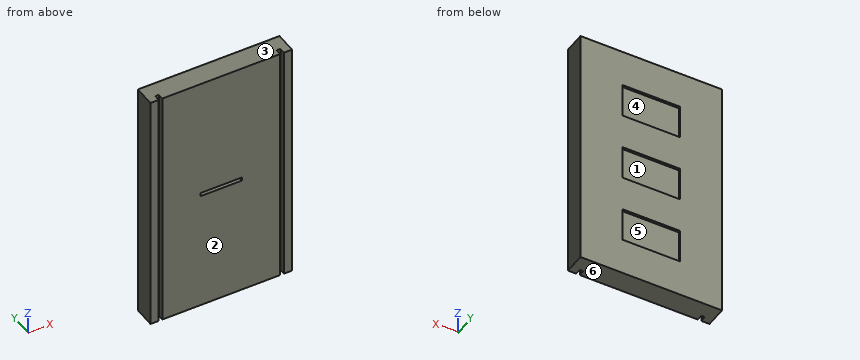
Autodesk Inventor part; units mm, degrees
ref_plane "YZ Plane" through (0, 0, 0) normal (1, 0, 0) x (0, 1, 0)
ref_plane "XZ Plane" through (0, 0, 0) normal (0, 1, 0) x (-1, 0, 0)
ref_plane "XY Plane" through (0, 0, 0) normal (0, 0, 1) x (1, 0, 0)
sketch "Sketch1" plane through (0, 0, 0) normal (0, 0, 1) x (1, 0, 0)
  line L0 (0, 0) -> (120, 0)
  line L1 (120, 0) -> (120, 18)
  line L2 (120, 18) -> (0, 18)
  line L3 (0, 18) -> (0, 0)
  dimension "d0" = 18
  dimension "d1" = 120
extrude "Extrusion1" add sketch "Sketch1" along normal blind 210
sketch "Sketch2" plane through (0, 0, 210) normal (0, 0, 1) x (1, 0, 0)
  line L0 (0, 0) -> (120, 0)
  line L1 (7, 0) -> (10, 0)
  line L2 (10, 0) -> (10, 5)
  line L3 (10, 5) -> (7, 5)
  line L4 (7, 5) -> (7, 0)
  line L5 (60, 0) -> (60, -17.5294) construction
  line L6 (113, 0) -> (110, 0)
  line L7 (110, 0) -> (110, 5)
  line L8 (110, 5) -> (113, 5)
  line L9 (113, 5) -> (113, 0)
  point P0 (110, 0)
  point P1 (113, 0)
  dimension "d4" = 3
  dimension "d5" = 5
  dimension "d26" = 100
extrude "Extrusion2" cut sketch "Sketch2" against normal through all
sketch "Sketch3" plane through (0, 18, 0) normal (0, 1, 0) x (1, 0, 0)
  line L0 (35.5, -31.5) -> (84.5, -31.5)
  line L1 (84.5, -31.5) -> (84.5, -60.5)
  line L2 (84.5, -60.5) -> (35.5, -60.5)
  line L3 (35.5, -60.5) -> (35.5, -31.5)
  line L4 (35.5, -90.5) -> (84.5, -90.5)
  line L5 (84.5, -90.5) -> (84.5, -119.5)
  line L6 (84.5, -119.5) -> (35.5, -119.5)
  line L7 (35.5, -119.5) -> (35.5, -90.5)
  line L8 (35.5, -149.5) -> (84.5, -149.5)
  line L9 (84.5, -149.5) -> (84.5, -178.5)
  line L10 (84.5, -178.5) -> (35.5, -178.5)
  line L11 (35.5, -178.5) -> (35.5, -149.5)
  line L12 (0, 0) -> (0, -210)
  line L13 (120, 0) -> (0, 0)
  point P0 (0, -105)
  point P1 (35.5, -105)
  point P2 (60, 0)
  point P3 (60, -31.5)
  dimension "d9" = 29
  dimension "d10" = 49
  dimension "d13" = 59
extrude "Extrusion3" cut sketch "Sketch3" against normal blind 2
sketch "Sketch4" plane through (10, 0, 0) normal (0, -1, 0) x (1, 0, 0)
  line L0 (-10, 0) -> (-10, 210)
  line L1 (0, 0) -> (100, 0)
  line L2 (32.5, 106.5) -> (67.5, 106.5)
  line L3 (67.5, 106.5) -> (67.5, 103.5)
  line L4 (67.5, 103.5) -> (32.5, 103.5)
  line L5 (32.5, 103.5) -> (32.5, 106.5)
  point P0 (-10, 105)
  point P1 (32.5, 105)
  point P2 (50, 103.5)
  point P3 (50, 0)
  dimension "d20" = 3
  dimension "d21" = 35
extrude "Extrusion4" cut sketch "Sketch4" against normal blind 5
properties part number "topplatform"
Design review of the part built by this model. Coordinates are the model's own, in mm. Face numbers are marked on the shaded views. A direction names the side the tool comes from. Round coordinates to 2 decimals unless told otherwise and drop trailing zeros. Order: outer loops, then holes, each group sorted by start corner. A loop starts at its lowest first (then second) coordinate and runs counter-clockwise, first axis right, second up. Notation, with made-up numbers: (15, 22.5) - (26, 22.5) arc R22 ccw to (26, 37.5) - close; hole circle Ø9 at (-22, 38.5). An arc over 180 degrees is marked (long way). Return JSON: item names as keys, results as strings.
Q1. Machinability: for the marked faces 5 and 6, which of the approach directions +Z, -Z, +X, -X, +Y, -Y give a long, thin tool a straight path to every point of the face, cutting with its end or side? Answer none if there is none.
Computed values:
{"face 5": "+Y", "face 6": "-Z, +X, -X, +Y, -Y"}
Q2. Consider section C-C on z = 55. Write out the cut boundary in (x, y).
Computed values:
{"outline": "(0, 0) - (7, 0) - (7, 5) - (10, 5) - (10, 0) - (110, 0) - (110, 5) - (113, 5) - (113, 0) - (120, 0) - (120, 18) - (84.5, 18) - (84.5, 16) - (35.5, 16) - (35.5, 18) - (0, 18) - close"}
Q3. Wall thickness on L1, parallel to X at y = 4.25, z = 92.5; L2, parallel to Z at x = 79.5, y = 16.5; L3, parallel to Z at x = 67, y = 1: over which ranges is each line inside the solid? List them lowest first. Write a range as [from, to].
Computed values:
{"L1": "x = [0, 7], [10, 110], [113, 120]", "L2": "z = [0, 31.5], [60.5, 90.5], [119.5, 149.5], [178.5, 210]", "L3": "z = [0, 103.5], [106.5, 210]"}
Q4. Consider section B-B on x = 65.5. Write out the cut boundary in (y, z).
Computed values:
{"outline": "(0, 0) - (18, 0) - (18, 31.5) - (16, 31.5) - (16, 60.5) - (18, 60.5) - (18, 90.5) - (16, 90.5) - (16, 119.5) - (18, 119.5) - (18, 149.5) - (16, 149.5) - (16, 178.5) - (18, 178.5) - (18, 210) - (0, 210) - (0, 106.5) - (5, 106.5) - (5, 103.5) - (0, 103.5) - close"}
Q5. Consider section A-A on y = 2.75. Write out the cut boundary in (x, z), plus the area to 3 significant figures.
Computed values:
{"outline": "(0, 0) - (7, 0) - (7, 210) - (0, 210) - close; (10, 0) - (110, 0) - (110, 210) - (10, 210) - close; (113, 0) - (120, 0) - (120, 210) - (113, 210) - close; hole (42.5, 103.5) - (77.5, 103.5) - (77.5, 106.5) - (42.5, 106.5) - close", "area": "23,800 mm2"}
Q6. Consider section D-D on x = 38. Write out the cut boundary in (y, z).
Computed values:
{"outline": "(0, 0) - (18, 0) - (18, 31.5) - (16, 31.5) - (16, 60.5) - (18, 60.5) - (18, 90.5) - (16, 90.5) - (16, 119.5) - (18, 119.5) - (18, 149.5) - (16, 149.5) - (16, 178.5) - (18, 178.5) - (18, 210) - (0, 210) - close"}
Q7. For pin 1 Ø8.5 at (x, z) = (52.5, 102.5) entering from +Y, flat-tipped, find the tip position at first contact; note if it passes through.
Computed values:
{"pin 1": "stops at y = 16"}
Q8. The part is to be moulded in two halves that separate along Z. For the marked faces 1, 2, 3 and 4, say which applies: pulls with the +Z half, pulls with the -Z half, needs draft (parallel to the pull), parting line crosses it, or undercut.
Computed values:
{"face 1": "undercut", "face 2": "needs draft", "face 3": "pulls with the +Z half", "face 4": "undercut"}
